Could you check a few things on this model? Use its own coordinates, in mm. Give positions to 0.01 mm unless a question says otherwise; leave off trailing zeros. Write each loop counter-clockwise with the first axis right and the second up, starting at its lowest first coordinate (ties: lowest second). Pieces come first, ordered by that corner, then holes. Notation, with made-up numbers: (46.5, 73) - (50.5, 73) arc R34 cw to (50.5, 110) - close; hole circle Ø11 at (56.5, 51). An arc over 180 degrees is marked (long way). Use one line per item in the form item = value.
```python
from build123d import *

# Parameters (mm, degrees)
BOSS_EXTRUDE1_DEPTH = 1.3
SKETCH3_W           = 100
SKETCH3_H           = 100
BOSS_EXTRUDE3_DEPTH = 1.3
SKETCH2_R           = 1.95
CUT_EXTRUDE1_DEPTH  = 1.3


with BuildPart() as part:
    # Sketch1 → Boss-Extrude1 (new body)
    with BuildSketch(Plane(origin=(0, 0, 0), x_dir=(1, 0, 0), z_dir=(0, 1, 0))):
        Polygon((7.2, 7.2), (7.2, 0), (90.2, 0), (90.2, 7.2), (97.4, 7.2), (97.4, 90.2), (90.2, 90.2), (90.2, 97.4), (7.2, 97.4), (7.2, 90.2), (0, 90.2), (0, 7.2), align=None)
    extrude(amount=BOSS_EXTRUDE1_DEPTH)

    # Sketch3 → Boss-Extrude3 (add)
    with BuildSketch(Plane(origin=(0, 1.3, 0), x_dir=(1, 0, 0), z_dir=(0, 1, 0))):
        with Locations((48.7, 48.7)):
            Rectangle(SKETCH3_W, SKETCH3_H)
    extrude(amount=-BOSS_EXTRUDE3_DEPTH)

    # Sketch2 → Cut-Extrude1 (cut)
    with BuildSketch(Plane.XZ):
        with Locations(Location((92.4, -86.3, 0), (0, 0, 270))):
            Circle(SKETCH2_R)
        with Locations(Location((86.3, -92.4, 0), (0, 0, 270))):
            Circle(SKETCH2_R)
        with Locations(Location((11.1, -92.4, 0), (0, 0, 270))):
            Circle(SKETCH2_R)
        with Locations(Location((5, -86.3, 0), (0, 0, 270))):
            Circle(SKETCH2_R)
        with Locations(Location((5, -11.1, 0), (0, 0, 270))):
            Circle(SKETCH2_R)
        with Locations(Location((11.1, -5, 0), (0, 0, 270))):
            Circle(SKETCH2_R)
        with Locations(Location((86.3, -5, 0), (0, 0, 270))):
            Circle(SKETCH2_R)
        with Locations(Location((92.4, -11.1, 0), (0, 0, 270))):
            Circle(SKETCH2_R)
    extrude(amount=-CUT_EXTRUDE1_DEPTH, mode=Mode.SUBTRACT)


solid = part.part
```
1. Imagine slicing it at B-B, the plane x = 92.4. List the corners of the cut face in (y, z) for me.
Response values:
outline = (0, -98.7) - (1.3, -98.7) - (1.3, -88.25) - (0, -88.25) - close; (0, -84.35) - (1.3, -84.35) - (1.3, -13.05) - (0, -13.05) - close; (0, -9.15) - (1.3, -9.15) - (1.3, 1.3) - (0, 1.3) - close
2. If we mould it in two halves opening along X, with no side actions, what happens to faces 1 (the face through (93.718, 0.641, -84.863)), 2 (the face through (48, 0, -49))? For each: pulls with the +X half, pulls with the -X half, needs draft (parallel to the pull), parting line crosses it, or undercut.
Response values:
face_1 = undercut
face_2 = needs draft
3. Imagine slicing it at A-A, the plane z = -86.3. List the corners of the cut face in (x, y) for me, and give its area (3 significant figures).
Response values:
outline = (-1.3, 0) - (3.05, 0) - (3.05, 1.3) - (-1.3, 1.3) - close; (6.95, 0) - (90.45, 0) - (90.45, 1.3) - (6.95, 1.3) - close; (94.35, 0) - (98.7, 0) - (98.7, 1.3) - (94.35, 1.3) - close
area = 120 mm²
4. If I drill on line 1 (X direction, y = 0.8, z = -5); line 2 (X direction, y = 0.6, z = -11.1); line 3 (Z direction, x = 85, y = 0.6), over which ranges is the centre line in solid material (lowest first)? Write a range as from..to.
Response values:
line_1 = -1.3..9.15, 13.05..84.35, 88.25..98.7
line_2 = -1.3..3.05, 6.95..90.45, 94.35..98.7
line_3 = -98.7..-93.85, -90.95..-6.45, -3.55..1.3
